Autodesk Inventor part; units mm, degrees
ref_plane "YZ Plane" through (0, 0, 0) normal (1, 0, 0) x (0, 1, 0)
ref_plane "XZ Plane" through (0, 0, 0) normal (0, 1, 0) x (-1, 0, 0)
ref_plane "XY Plane" through (0, 0, 0) normal (0, 0, 1) x (1, 0, 0)
sketch "Sketch1" plane through (0, 0, 0) normal (1, 0, 0) x (0, 1, 0)
  line L0 (-15, 15) -> (15, 15)
  line L1 (15, 15) -> (15, -15)
  line L2 (15, -15) -> (-15, -15)
  line L3 (-15, -15) -> (-15, 15)
  line L4 (-15, 15) -> (15, -15) construction
  line L5 (15, 15) -> (-15, -15) construction
  point P0 (0, 0)
  dimension "d0" = 30
  dimension "d1" = 30
extrude "Extrusion1" add sketch "Sketch1" along normal blind 50
sketch "Sketch2" plane through (50, 0, 0) normal (1, 0, 0) x (0, 0, -1)
  circle A0 centre (0, 0) radius 3.9
  dimension "d5" = 7.8
extrude "Extrusion2" add sketch "Sketch2" along normal blind 20 and the other way blind 70
sketch "Sketch3" plane through (0, 15, 15) normal (0, 1, 0) x (1, 0, 0)
  line L0 (16.5, 30) -> (33.5, 30)
  line L1 (33.5, 30) -> (33.5, 0)
  line L2 (33.5, 0) -> (16.5, 0)
  line L3 (16.5, 0) -> (16.5, 30)
  line L4 (16.5, 30) -> (33.5, 0) construction
  line L5 (33.5, 30) -> (16.5, 0) construction
  point P0 (0, 15)
  point P1 (25, 15)
  dimension "d10" = 17
  dimension "d11" = 30
extrude "Extrusion3" add sketch "Sketch3" along normal blind 40
sketch "Sketch4" plane through (0, -15, -15) normal (0, -1, 0) x (1, 0, 0)
  point P0 (0, 15)
sketch "Sketch5" plane through (0, -15, 15) normal (0, 0, 1) x (1, 0, 0)
  line L0 (0, 15) -> (50, 15)
  line L1 (50, 30) -> (50, 0)
  circle A0 centre (25, 15) radius 5
  dimension "d14" = 10
extrude "Extrusion4" cut sketch "Sketch5" against normal through all
sketch "Sketch6" plane through (0, -15, -15) normal (0, 0, -1) x (-1, 0, 0)
  point P0 (0, 15)
sketch "Sketch7" plane through (0, -15, 15) normal (0, 0, 1) x (1, 0, 0)
  circle A0 centre (25, 15) radius 5
  circle A1 centre (25, 15) radius 11.35
  point P0 (0, 15)
  dimension "d17" = 22.7
extrude "Extrusion5" cut sketch "Sketch7" against normal blind 4
sketch "Sketch8" plane through (0, 55, 15) normal (0, 1, 0) x (1, 0, 0)
  line L0 (16.5, 0) -> (16.5, 30)
  line L1 (16.5, 0) -> (33.5, 0)
  line L2 (16.5, 30) -> (33.5, 0)
  line L3 (33.5, 30) -> (33.5, 0)
  line L4 (16.5, 22.5) -> (33.5, 22.5)
  line L5 (33.5, 22.5) -> (33.5, 7.5)
  line L6 (33.5, 7.5) -> (16.5, 7.5)
  line L7 (16.5, 7.5) -> (16.5, 22.5)
  line L8 (16.5, 22.5) -> (33.5, 7.5) construction
  line L9 (33.5, 22.5) -> (16.5, 7.5) construction
  point P0 (0, 15)
  point P1 (25, 15)
  dimension "d20" = 15
extrude "Extrusion6" cut sketch "Sketch8" against normal blind 25 contours L0 L4 L2 L6 | L2 L4 L3 L6
sketch "Sketch9" plane through (16.5, 55, -7.5) normal (0, 0, 1) x (1, 0, 0)
  line L0 (17, 0) -> (0, 0)
  line L1 (8.5, 0) -> (8.5, -25)
  line L2 (8.5, 0) -> (8.5, -7)
  line L3 (8.5, -7) -> (8.5, -25)
  line L4 (8.5, -25) -> (8.5, -20)
  circle A0 centre (8.5, -7) radius 3.5
  circle A1 centre (8.5, -20) radius 3.5
  point P0 (-16.5, -55)
  dimension "d23" = 25
  dimension "d24" = 7
  dimension "d25" = 5
  dimension "d26" = 7
  dimension "d27" = 7
extrude "Extrusion7" cut sketch "Sketch9" along normal mid plane 100
sketch "Sketch10" plane through (0, -15, 15) normal (0, 0, 1) x (1, 0, 0)
  circle A0 centre (25, 63) radius 3.5
  line L0 (30.7735, 63) -> (27.8868, 58)
  line L1 (27.8868, 58) -> (22.1132, 58)
  line L2 (22.1132, 58) -> (19.2265, 63)
  line L3 (19.2265, 63) -> (22.1132, 68)
  line L4 (22.1132, 68) -> (27.8868, 68)
  line L5 (27.8868, 68) -> (30.7735, 63)
  circle A1 centre (25, 50) radius 3.5
  line L6 (30.7735, 50) -> (27.8868, 45)
  line L7 (27.8868, 45) -> (22.1132, 45)
  line L8 (22.1132, 45) -> (19.2265, 50)
  line L9 (19.2265, 50) -> (22.1132, 55)
  line L10 (22.1132, 55) -> (27.8868, 55)
  line L11 (27.8868, 55) -> (30.7735, 50)
  point P0 (0, 15)
  dimension "d30" = 10
  dimension "d31" = 10
extrude "Extrusion8" cut sketch "Sketch10" against normal blind 5
sketch "Sketch11" plane through (0, -15, -15) normal (0, 0, -1) x (-1, 0, 0)
  circle A0 centre (-25, 63) radius 3.5
  circle A1 centre (-25, 63) radius 5.25
  circle A2 centre (-25, 50) radius 3.5
  circle A3 centre (-25, 50) radius 5.25
  point P0 (0, 15)
  dimension "d34" = 10.5
  dimension "d35" = 10.5
extrude "Extrusion9" cut sketch "Sketch11" against normal blind 3 contours A0 | A1 | A2 | A3
properties part number "L0wer_battery"
Could you check a few things on this model? Use its own coordinates, in mm. A direction names the side the tool comes from. Coordinates: 2 decimals unless noted, no trailing zeros. Write each loop counter-clockwise with the first axis right and the second up, starting at its lowest first coordinate (ties: lowest second). Pieces come first, ordered by that corner, then holes. Notation, with made-up numbers: M 65,37.25 L 94,37.25 A24 ccw 94,52.25 Z; hole C 26,31.5 d9. An arc over 180 degrees is marked long. One line per question, with ' | ' between items.
1) For faces 4 (the face through (25, 30, 0)), 5 (the face through (50, -4, 4)), 6 (the face through (35.826, 3.409, 13.028)), which set-ups out of +Z, -Z, +X, -X, +Y, -Y let a thin tool reach every point of the face, with its end or its side?
Checks:
face 4: +X, -X, +Y | face 5: +X | face 6: +Z
2) Imagine slicing it at D-D, the plane x = 25. Give the number of separate pieces and of enclosed holes in the cut face, and give its area (3 significant figures).
Checks:
separate pieces: 6 | enclosed holes: 0 | area: 1,110 mm²
3) For pin 1 Ø13.5 at (x, y) = (25, 0) entering from -Z; pin 2 Ø10 at (y, z) = (7, -9.5) entering from +X; pin 3 Ø7 at (x, y) = (27, 1.5) entering from +Z; pin 4 Ø8 at (y, z) = (44.5, -9) entering from -X, each with a flat end and sliding along its axis, tell me the tip position at first contact or that it passes through.
Checks:
pin 1: z = -15 | pin 2: x = 50 | pin 3: z = 11 | pin 4: x = 16.5
4) If we mould it in two halves opening along Y, with no side actions, what happens to faces 1 (the face through (0, -4, 4)), 2 (the face through (25, 43, 13)), 3 (the face through (25, 55, 11))? For each: released by +Y, released by -Y, zero draft, split by the parting line, or undercut.
Checks:
face 1: zero draft | face 2: undercut | face 3: released by +Y
5) Imagine slicing it at A-A, the plane z = -1.5. Write out the boundary of the cut face in (x, y).
Checks:
outline: M -20,-3.6 L 0,-3.6 L 0,-15 L 50,-15 L 50,-3.6 L 70,-3.6 L 70,3.6 L 50,3.6 L 50,15 L 33.5,15 L 33.5,30 L 16.5,30 L 16.5,15 L 0,15 L 0,3.6 L -20,3.6 Z; hole C 25,0 d10
6) Imagine slicing it at C-C, the plane z = -10.75. Write out the boundary of the cut face in (x, y), and give its area (3 significant figures).
Checks:
outline: M 0,-15 L 50,-15 L 50,15 L 33.5,15 L 33.5,55 L 16.5,55 L 16.5,15 L 0,15 Z; hole C 25,0 d10; hole C 25,35 d7; hole C 25,48 d7 | area: 2,020 mm²
7) Imagine slicing it at B-B, the plane y = 0. Write out the boundary of the cut face in (x, z).
Checks:
outline: M -20,-3.9 L 0,-3.9 L 0,-15 L 20,-15 L 20,11 L 13.65,11 L 13.65,15 L 0,15 L 0,3.9 L -20,3.9 Z; M 30,-15 L 50,-15 L 50,-3.9 L 70,-3.9 L 70,3.9 L 50,3.9 L 50,15 L 36.35,15 L 36.35,11 L 30,11 Z
8) I need wall thicknesses on probe 1 along Y at (x, z) = (25, -10.9); probe 2 along Y at (x, z) = (25, -12.85); probe 3 along Y at (x, z) = (25, 3). Which ranges of each line are inside material? Lowest first, please. Write a range as [from, to].
Checks:
probe 1: [-15, -5], [5, 31.5], [38.5, 44.5], [51.5, 55] | probe 2: [-15, -5], [5, 29.75], [40.25, 42.75], [53.25, 55] | probe 3: [-15, -5], [5, 30]
